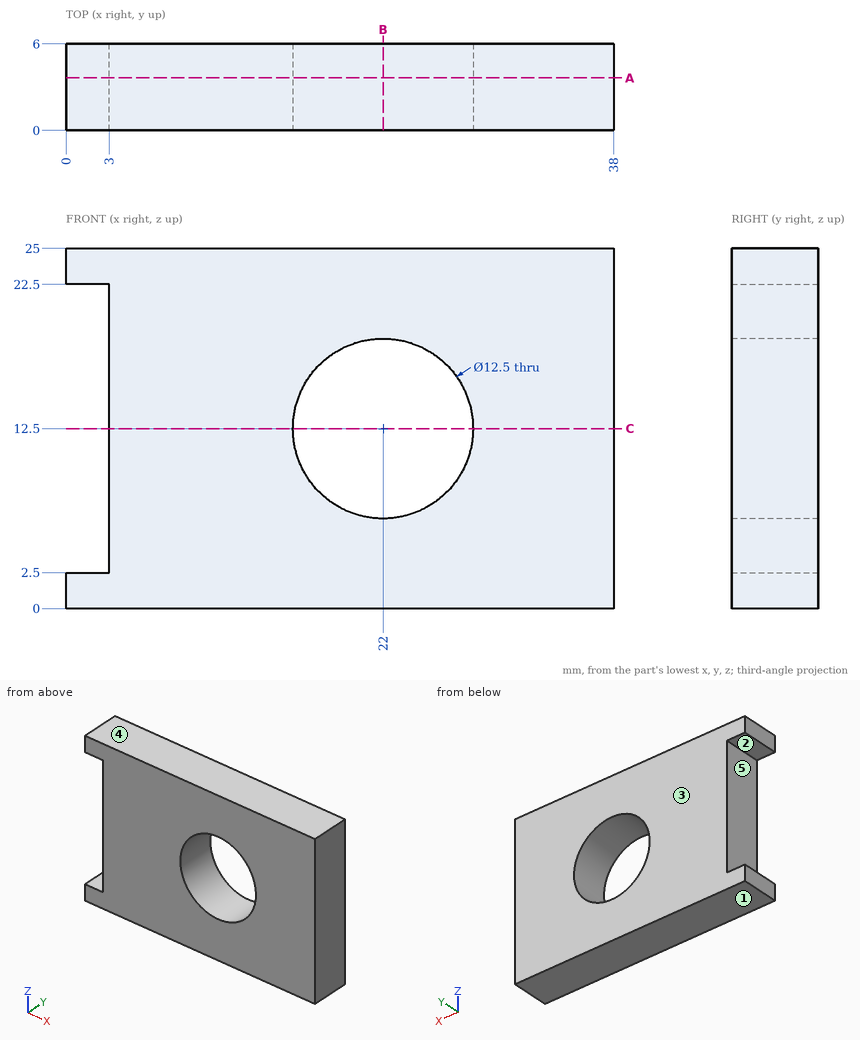
Study the drawing (mm; zero at the part's minimum x, y, z) and answer. A direction names the side the tool comes from. Round coordinates to 2 decimals unless told otherwise and drop trailing zeros. Loops run counter-clockwise (first coordinate to the right, second up) from the corner with the lowest first, then second, coordinate; pieces in that order, holes last. Notation, with made-up numbers: (26.25, 32) -> (79.25, 32) arc R11 cw to (79.25, 51) -> close; hole circle Ø6 at (-18, 23). An arc over 180 degrees is marked (long way). Write each question's results on one line, items separated by ' | '. Start each with the question number.
1. Section A-A (y = 3.65) is taken. Determine the outline of the cut face in (x, z), plus the area to 3 significant figures.
2. Given pin 1 Ø10 at (x, z) = (22, 12.5) entering from -Y, flat-ended and moving along its own axis, determine where the tip first touches the part or whether it passes through.
3. Section C-C (z = 12.5) is taken. Determine the outline of the cut face in (x, y).
4. For a pull along Z with two mould halves and no side action, classify the marked faces 3, 4 and 5 as +Z half, -Z half, draft (parallel to the pull), parting line (faces both ways), or undercut.
5. Find the intervals of material crossed by probe 1 along X at (y, z) = (2.8, 12.25) (3 decimals); probe 2 along Z at (x, y) = (2.5, 2.55); probe 3 along X at (y, z) = (5.35, 20.25), in increasing order. Write a range as from..to.
6. A tool of negligible diameter and unlimited length cuts with its end or side. For the marked faces 1 and 2, from which of +Z, -Z, +X, -X, +Y, -Y can it reach the whole face along a straight path? Write none if from no direction.
7. Section B-B (x = 22) is taken. Determine the outline of the cut face in (y, z), plus the area to 3 significant figures.
Evaluation:
1) outline: (0, 0) -> (38, 0) -> (38, 25) -> (0, 25) -> (0, 22.5) -> (3, 22.5) -> (3, 2.5) -> (0, 2.5) -> close; hole circle Ø12.5 at (22, 12.5) | area: 767 mm2
2) pin 1: passes through
3) outline: (3, 0) -> (15.75, 0) -> (15.75, 6) -> (3, 6) -> close; (28.25, 0) -> (38, 0) -> (38, 6) -> (28.25, 6) -> close
4) face 3: draft | face 4: +Z half | face 5: undercut
5) probe 1: x = 3..15.755, 28.245..38 | probe 2: z = 0..2.5, 22.5..25 | probe 3: x = 3..38
6) face 1: -Z, +X, -X, +Y, -Y | face 2: -X, +Y, -Y
7) outline: (0, 0) -> (6, 0) -> (6, 6.25) -> (0, 6.25) -> close; (0, 18.75) -> (6, 18.75) -> (6, 25) -> (0, 25) -> close | area: 75.0 mm2
